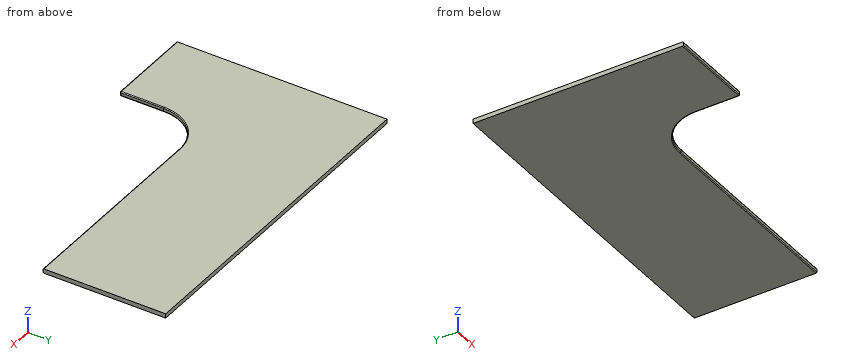
```python
from build123d import *

# Parameters (mm, degrees)
F1_DEPTH = 25
F2_R     = 5


with BuildPart() as f1:
    # F0 (on Top) → F1 (new body)
    with BuildSketch(Plane.XY):
        with BuildLine():
            Line((0, 0), (0, -1200))
            Line((0, -1200), (500, -1200))
            Line((500, -1200), (500, -950))
            ThreePointArc((500, -950), (573.223305, -773.223305), (750, -700))
            Line((750, -700), (1950, -700))
            Line((1950, -700), (1950, 0))
            Line((1950, 0), (0, 0))
        make_face()
    extrude(amount=F1_DEPTH)

    # F2
    f2_edges = [f1.edges().sort_by_distance(p)[0] for p in [
        (1350, -700, 25),
        (1350, -700, 0),
        (250, -1200, 25),
        (250, -1200, 0),
        (500, -1200, 12.5),
    ]]
    fillet(f2_edges, radius=F2_R)


solid = f1.part
```
The listing builds one solid part. Answer for the finished solid, in the listing's coordinates (mm). Round coordinates to 2 decimals unless told otherwise and drop trailing zeros. Loops run counter-clockwise (first coordinate to the right, second up) from the corner with the lowest first, then second, coordinate; pieces in that order, holes last. Notation, with made-up numbers: (70.25, -11) - (109.25, -11) arc R11 ccw to (109.25, -2) - close; hole circle Ø2 at (56, 23). An arc over 180 degrees is marked (long way). Use one line per item in the form item = value. Start each with the question number.
1. Consider line 1 (Y direction, x = 293, z = 21.5); line 2 (Y direction, x = 892.5, z = 16); line 3 (X direction, y = -955, z = 19.75). Determine where each line is inside the solid, lowest interval first. Write a range as [from, to].
2. The part is cut by section B-B on x = 1055.5. Determine the outline of the cut face in (y, z).
3. The part is cut by section A-A on z = 15.75. Determine the outline of the cut face in (x, y), then the cut area to 3 significant figures.
4. Given pin 1 Ø12 at (y, z) = (-1102.5, 14.5) entering from +X; pin 2 Ø1.5 at (x, z) = (1258.5, 3) entering from -Y; pin 3 Ø1.5 at (x, z) = (1565, 20) entering from -Y, each flat-ended and moving along its own axis, determine where each tip first touches the part or whether it passes through.
Geometry check:
q1.line_1 = [-1199.77, 0]
q1.line_2 = [-700, 0]
q1.line_3 = [0, 500]
q2.outline = (-700, 5) arc R5 ccw to (-695, 0) - (0, 0) - (0, 25) - (-695, 25) arc R5 ccw to (-700, 20) - close
q3.outline = (0, -1200) - (495, -1200) arc R5 ccw to (500, -1195) - (500, -950) arc R250 cw to (750, -700) - (1950, -700) - (1950, 0) - (0, 0) - close
q3.area = 1,630,000 mm^2
q4.pin_1 = 500
q4.pin_2 = -699.84
q4.pin_3 = -700
